Autodesk Inventor part; units mm, degrees
ref_plane "РабПлоскость1" through (0, 80, 0) normal (0, 1, 0) x (-1, 0, 0)
ref_plane "YZ Plane" through (0, 0, 0) normal (1, 0, 0) x (0, 1, 0)
ref_plane "XY Plane" through (0, 0, 0) normal (0, 0, 1) x (1, 0, 0)
sketch "Эскиз1" plane through (0, 0, 0) normal (0, 1, 0) x (-1, 0, 0)
  line L0 (-30, 0) -> (-30, -30)
  line L1 (-30, 0) -> (-30, 30)
  circle A0 centre (0, 35) radius 10
  arc A1 (20, 35) -> (-20, 35) centre (0, 35) ccw
  line L2 (-25, 35) -> (-30, 30)
  circle A2 centre (0, -35) radius 10
  arc A3 (-20, -35) -> (20, -35) centre (0, -35) ccw
  line L3 (-30, -30) -> (-25, -35)
  line L4 (30, 30) -> (30, -30)
  line L5 (25, 35) -> (30, 30)
  line L6 (25, -35) -> (30, -30)
  line L7 (-25, 35) -> (-20, 35)
  line L8 (20, 35) -> (25, 35)
  line L9 (-25, -35) -> (-20, -35)
  line L10 (20, -35) -> (25, -35)
  point P0 (0, 0)
  point P1 (-30, -35)
  point P2 (-30, 35)
  point P3 (30, 35)
  point P4 (30, -35)
  point P5 (30, 35)
  point P6 (30, -35)
  dimension "d0" = 35
  dimension "d1" = 35
  dimension "d2" = 20
  dimension "d3" = 40
  dimension "d4" = 5
  dimension "d5" = 5
  dimension "d6" = 20
  dimension "d7" = 40
  dimension "d8" = 5
  dimension "d9" = 5
  dimension "d10" = 5
  dimension "d11" = 5
  dimension "d12" = 5
  dimension "d13" = 5
extrude "Выдавливание1" add sketch "Эскиз1" along normal blind 20
sketch "Эскиз2" plane through (0, 20, 0) normal (0, 1, 0) x (1, 0, 0)
  line L0 (20, 20) -> (-20, 20)
  line L1 (-20, 20) -> (-20, -20)
  line L2 (-20, -20) -> (20, -20)
  line L3 (20, -20) -> (20, 20)
  line L4 (20, 20) -> (-20, -20) construction
  line L5 (-20, 20) -> (20, -20) construction
  point P0 (0, 0)
  dimension "d16" = 40
  dimension "d17" = 40
extrude "Выдавливание2" add sketch "Эскиз2" along normal blind 20
sketch "Эскиз3" plane through (0, 40, 0) normal (0, 1, 0) x (1, 0, 0)
  line L0 (-7, -20) -> (-7, 20)
  line L1 (-7, -20) -> (-20, -20)
  line L2 (-20, -20) -> (-20, 20)
  line L3 (7, -20) -> (7, 20)
  line L4 (20, -20) -> (7, -20)
  line L5 (-7, -20) -> (-20, -20)
  line L6 (-20, 20) -> (-7, 20)
  line L7 (20, 20) -> (20, -20)
  line L8 (20, -20) -> (20, 20)
  line L9 (20, 20) -> (7, 20)
  point P0 (0, 0)
extrude "Выдавливание3" add sketch "Эскиз3" along normal blind 40
sketch "Эскиз4" plane through (20, 20, 20) normal (1, 0, 0) x (0, 0, -1)
  circle A0 centre (20, 45) radius 7
  point P0 (20, -20)
  dimension "d22" = 14
extrude "Выдавливание4" cut sketch "Эскиз4" against normal blind 40
ref_plane "РабПлоскость1" through (0, 80, 0) normal (0, 1, 0) x (-1, 0, 0)
sketch "Эскиз5" plane through (0, 80, 0) normal (0, 1, 0) x (-1, 0, 0)
  line L0 (0, 0) -> (-33, 0)
  line L1 (-33, 0) -> (-33, 61)
  line L2 (-33, 61) -> (0, 61)
  line L3 (0, 61) -> (0, 0)
extrude "Выдавливание5" cut sketch "Эскиз5" against normal blind 80
properties part number "пч2020"
Read the model definition and answer for the solid it produces. Units are mm, in the model's axes. A direction names the side the tool comes from. Coordinates: 2 decimals unless noted, no trailing zeros. Loops run counter-clockwise (first coordinate to the right, second up) from the corner with the lowest first, then second, coordinate; pieces in that order, holes last.
(1) Consider line 1 along Y through (x, z) = (-11, 0); line 2 along Z through (x, y) = (15.5, 36.5); line 3 along Y through (x, z) = (1.5, -23). Determine where each line is inside the solid, lowest interval first.
Solution:
line 1: y = 0 to 58, 72 to 80
line 2: z = -20 to 0
line 3: y = 0 to 20
(2) The part is cut by section D-D (z = -14). Determine the outline of the cut face in (x, y).
Solution:
outline: (-30, 0) - (30, 0) - (30, 20) - (20, 20) - (20, 80) - (7, 80) - (7, 40) - (-7, 40) - (-7, 80) - (-20, 80) - (-20, 20) - (-30, 20) - close
(3) The part is cut by section C-C (x = -3.5). Determine the outline of the cut face in (y, z).
Solution:
outline: (0, -54.69) - (20, -54.69) - (20, -44.37) - (0, -44.37) - close; (0, -25.63) - (20, -25.63) - (20, -20) - (40, -20) - (40, 20) - (20, 20) - (20, 25.63) - (0, 25.63) - close; (0, 44.37) - (20, 44.37) - (20, 54.69) - (0, 54.69) - close
(4) Flat-ended cylindrical pins translate along their axes: pin 1 Ø12 at (x, z) = (4, -35.5) entering from +Y; pin 2 Ø3 at (x, y) = (6, 64.5) entering from -Z; pin 3 Ø5.5 at (x, y) = (-23.5, 9) entering from +Z; pin 4 Ø11 at (y, z) = (65, 0) entering from +X. Find the tip coordinate at first contact, or state that the pin passes through.
Solution:
pin 1: stops at y = 20
pin 2: stops at z = -20
pin 3: stops at z = 35
pin 4: passes through
(5) The part is cut by section B-B (x = 4). Determine the outline of the cut face in (y, z), and give its area (3 significant figures).
Solution:
outline: (0, -54.6) - (20, -54.6) - (20, -44.17) - (0, -44.17) - close; (0, -25.83) - (20, -25.83) - (20, -20) - (40, -20) - (40, 0) - (0, 0) - close
area: 1,130 mm2
(6) The mould has two halves that part along X. Classify faces 1 (the face through (-27, 10, -33)), 2 (the face through (0, 20, 13)), 3 (the face through (-7, 55, 0)): released by +X, released by -X, zero draft, split by the parting line, or undercut.
Solution:
face 1: released by -X
face 2: released by +X
face 3: undercut
(7) A tool of negligible diameter and unlimited length cuts with its end or side. For faces 4 (the face through (-22, 10, -35)), 5 (the face through (-12, 50, 20)), 6 (the face through (11, 23, 0)), 7 (the face through (-9, 50, -20)), from which of +Z, -Z, +X, -X, +Y, -Y can it reach the whole face along a straight path? Write none if from no direction.
Solution:
face 4: -Z, -X, +Y, -Y
face 5: +Z, +X, -X, +Y
face 6: +Z, +X, +Y, -Y
face 7: -Z, +X, -X, +Y
(8) The part is cut by section A-A (y = 65). Determine the outline of the cut face in (x, z).
Solution:
outline: (-20, -20) - (-7, -20) - (-7, -7) - (-20, -7) - close; (-20, 7) - (-7, 7) - (-7, 20) - (-20, 20) - close; (7, -20) - (20, -20) - (20, -7) - (7, -7) - close
